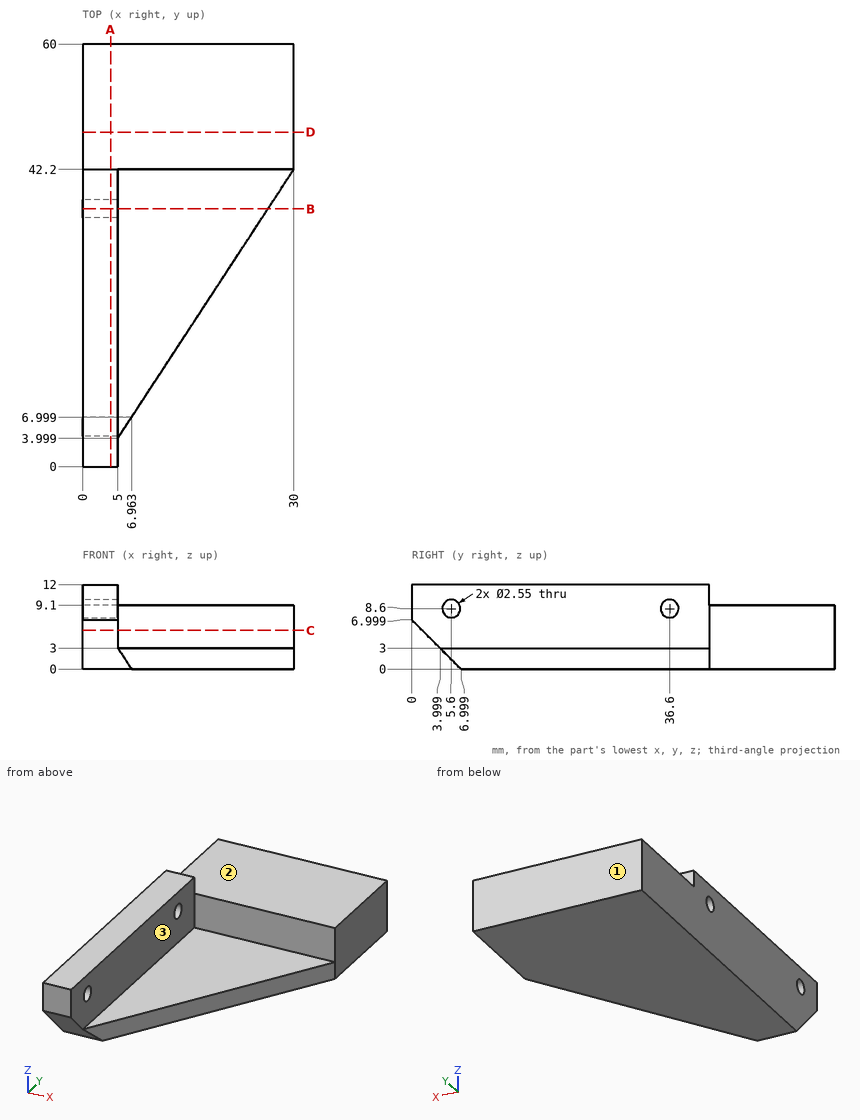
Here's the drawing with two shaded views (mm, measured from the low corner). I have some questions. A direction names the side the tool comes from. Round coordinates to 2 decimals unless told otherwise and drop trailing zeros. Write each loop counter-clockwise with the first axis right and the second up, starting at its lowest first coordinate (ties: lowest second). Pieces come first, ordered by that corner, then holes.
(1) Suppose I cut it at B-B on y = 36.6. Write out the boundary of the cut face in (x, z) (1 decimal).
Findings below:
outline: (0, 0) - (26.3, 0) - (26.3, 3) - (5, 3) - (5, 7.3) - (0, 7.3) - close; (0, 9.9) - (5, 9.9) - (5, 12) - (0, 12) - close
(2) Which directions (+Z, -Z, +X, -X, +Y, -Y) give clear straight access to the entire face, cutting with the end or side of a thin tool? Please do the marked faces 1, 2 and 3.
Findings below:
face 1: +Z, -Z, +X, -X, +Y
face 2: +Z, +X, -X, +Y
face 3: +Z, +X, -Y
(3) For pin 1 (5 mm diameter, centred on y = 34.5, z = 11, fed in from -X); pin 2 (12.5 mm diameter, centred on x = 20.5, y = 25, fed in from +Z); pin 3 (14 mm diameter, centred on x = 15.5, y = 55.5, fed in from +Z); pin 4 (7 mm diameter, centred on y = 15.5, z = 6, fed in from +X) (1 decimal), each with a flat end and sliding along its axis, tell me the tip position at first contact or that it passes through.
Findings below:
pin 1: stops at x = 0
pin 2: stops at z = 3
pin 3: stops at z = 9.1
pin 4: stops at x = 13.7
(4) Suppose I cut it at C-C on z = 5.5. Write out the boundary of the cut face in (x, y).
Findings below:
outline: (0, 1.5) - (5, 1.5) - (5, 42.2) - (30, 42.2) - (30, 60) - (0, 60) - close
(5) If I drill on probe 1 along Y at (x, z) = (2.7, 8.6) (1 decimal); probe 2 along Y at (x, z) = (26.5, 3.75); probe 3 along X at (y, z) = (18, 10), over which ranges is the centre line in solid material (lowest first)?
Findings below:
probe 1: y = 0 to 4.3, 6.9 to 35.3, 37.9 to 60
probe 2: y = 42.2 to 60
probe 3: x = 0 to 5
(6) Suppose I cut it at A-A on x = 4. State how many separate pieces and enclosed holes the cut face has, and give its area (3 significant figures).
Findings below:
separate pieces: 1
enclosed holes: 2
area: 634 mm2
(7) Suppose I cut it at D-D on y = 47.5. Write out the boundary of the cut face in (x, z), and give its area (3 significant figures).
Findings below:
outline: (0, 0) - (30, 0) - (30, 9.1) - (0, 9.1) - close
area: 273 mm2
